The figure shows three views and two pictorial views of one solid part (mm, origin at its lowest corner). Answer the questions. Coordinates: 2 decimals unless noted, no trailing zeros. Loops run counter-clockwise (first coordinate to the right, second up) from the corner with the lowest first, then second, coordinate; pieces in that order, holes last. Notation, with made-up numbers: (49.25, 3) -> (64.25, 3) arc R9 cw to (64.25, 8) -> close; hole circle Ø10 at (-7.75, -26.5). An arc over 180 degrees is marked (long way). Answer in a Markdown table with one row per item.
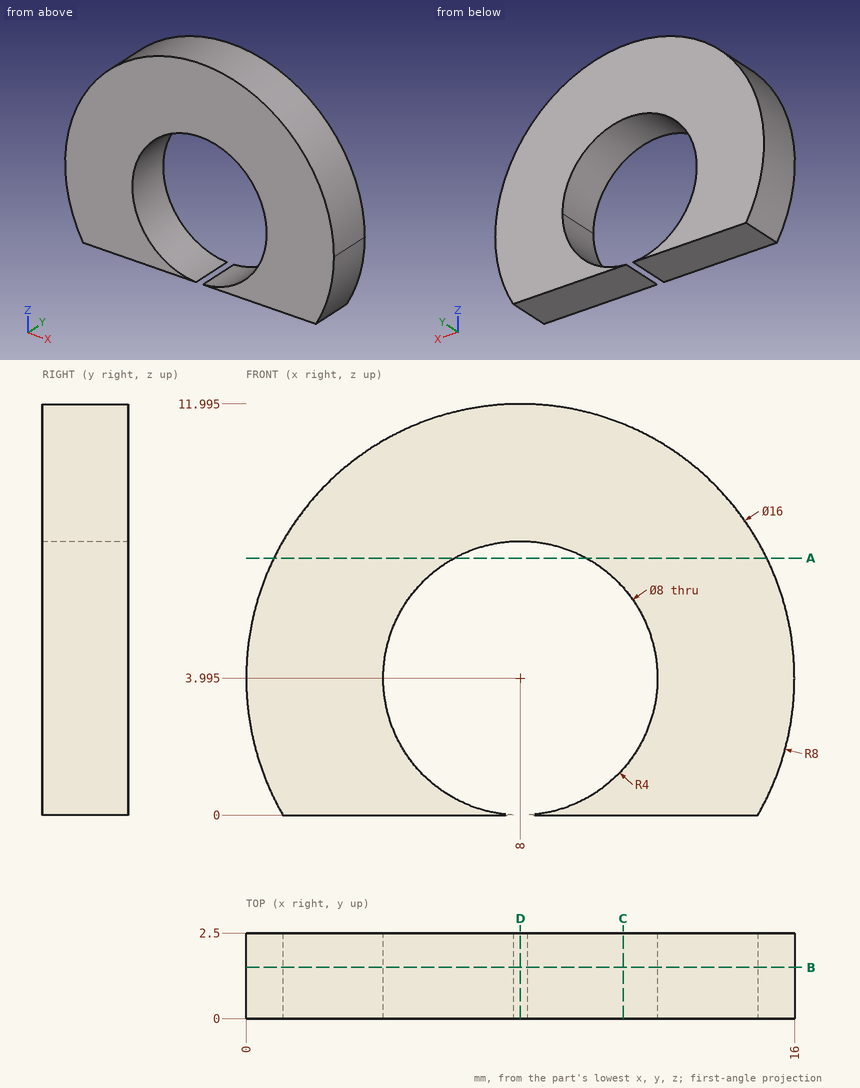
Item 1: A cutting plane is placed at A-A, the plane z = 7.5. Determine the outline of the cut face in (x, y), plus the area to 3 significant figures.
Findings below:
| item | result |
|---|---|
| outline | (0.81, 0) -> (6.07, 0) -> (6.07, 2.5) -> (0.81, 2.5) -> close; (9.93, 0) -> (15.19, 0) -> (15.19, 2.5) -> (9.93, 2.5) -> close |
| area | 26.3 mm2 |
Item 2: A cutting plane is placed at C-C, the plane x = 11. Determine the outline of the cut face in (y, z), plus the area to 3 significant figures.
Findings below:
| item | result |
|---|---|
| outline | (0, 0) -> (2.5, 0) -> (2.5, 1.35) -> (0, 1.35) -> close; (0, 6.64) -> (2.5, 6.64) -> (2.5, 11.41) -> (0, 11.41) -> close |
| area | 15.3 mm2 |
Item 3: A cutting plane is placed at B-B, the plane y = 1.5. Determine the outline of the cut face in (x, z) (3 decimals), plus the area to 3 significant figures.
Findings below:
| item | result |
|---|---|
| outline | (1.069, 0) -> (7.798, 0) arc R4 cw (long way) to (8.202, 0) -> (14.931, 0) arc R8 ccw (long way) to start |
| area | 111 mm2 |
Item 4: Flat-ended cylindrical pins translate along their axes: pin 1 Ø6.5 at (x, z) = (8, 3.99) entering from -Y; pin 2 Ø1 at (y, z) = (0.5, 8) entering from +X. Find the tip coordinate at first contact, or state that the pin passes through.
Findings below:
| item | result |
|---|---|
| pin 1 | passes through |
| pin 2 | stops at x = 15.19 |
Item 5: Find the intervals of material crossed by probe 1 along X at (y, z) = (0.15, 4); probe 2 along Z at (x, y) = (8, 1.3) (3 decimals); probe 3 along X at (y, z) = (2.2, 5), in increasing order.
Findings below:
| item | result |
|---|---|
| probe 1 | x = 0 to 4, 12 to 16 |
| probe 2 | z = 7.995 to 11.995 |
| probe 3 | x = 0.06 to 4.13, 11.87 to 15.94 |
Item 6: A cutting plane is placed at D-D, the plane x = 8. Determine the outline of the cut face in (y, z) (3 decimals).
Findings below:
| item | result |
|---|---|
| outline | (0, 7.995) -> (2.5, 7.995) -> (2.5, 11.995) -> (0, 11.995) -> close |
